Verification items for this drawing (mm, ordinates from the low corner). Give positions to 0.01 mm unless a question says otherwise; leave off trailing zeros. Order: outer loops, then holes, each group sorted by start corner. A loop starts at its lowest first (then second) coordinate and runs counter-clockwise, first axis right, second up.
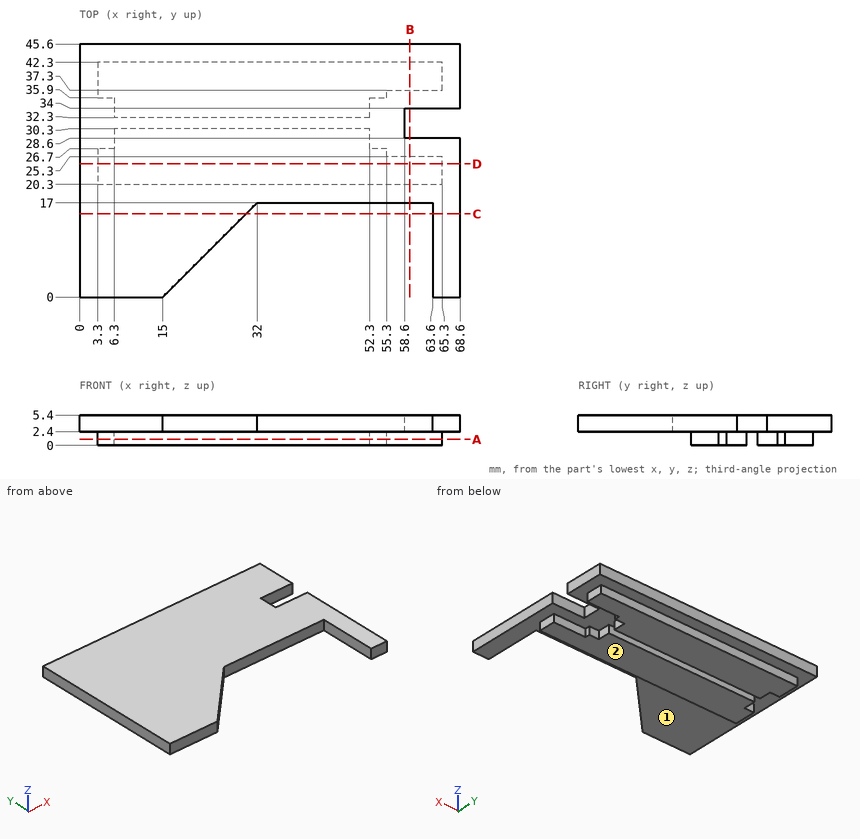
Q1. Release check for a two-part mould opening along Y. For the marked faces 1 and 2 record: pulls with the +Y half, pulls with the -Y half, needs draft (parallel to the pull), parting line crosses it, or undercut.
Q2. Cross-section at D-D, the plane y = 24. Record the boundary of the cut face in (x, z), and give its area (3 significant figures).
Q3. Cross-section at B-B, the plane x = 59.5. Record the boundary of the cut face in (y, z), and give its area (3 significant figures).
Q4. Cross-section at A-A, the plane z = 1.05. Record the boundary of the cut face in (x, y), and give its area (3 significant figures).
Q5. Thickness scan on L1, parallel to Y at x = 44, z = 2.1; L2, parallel to Y at x = 59.5, z = 1.55; L3, parallel to Z at x = 14.5, y = 10.5. Record the ranges inside material, lowest first.
Q6. Cross-section at C-C, the plane y = 15. Record the boundary of the cut face in (x, z), and give its area (3 significant figures).
Q7. Gauge pin test, flat ends, axial feed: P1, Ø8, axis at x = 38.5, y = 15.5, coming from the +Z side; P2, Ø1.2, axis at y = 22.5, z = 1.5, coming from the +X side; P3, Ø1, axis at x = 56, z = 3, coming from the -Y side; P4, Ø0.7, axis at x = 5.5, z = 1, coming from the +Y side. Record the tip position at first contact, or that the pin passes through.
Answers follow:
1. face 1: undercut
1. face 2: needs draft
2. outline: (0, 2.4) - (3.3, 2.4) - (3.3, 0) - (65.3, 0) - (65.3, 2.4) - (68.6, 2.4) - (68.6, 5.4) - (0, 5.4) - close
2. area: 355 mm2
3. outline: (17, 2.4) - (20.3, 2.4) - (20.3, 0) - (25.3, 0) - (25.3, 2.4) - (28.6, 2.4) - (28.6, 5.4) - (17, 5.4) - close; (34, 2.4) - (37.3, 2.4) - (37.3, 0) - (42.3, 0) - (42.3, 2.4) - (45.6, 2.4) - (45.6, 5.4) - (34, 5.4) - close
3. area: 93.6 mm2
4. outline: (3.3, 20.3) - (65.3, 20.3) - (65.3, 25.3) - (55.3, 25.3) - (55.3, 26.7) - (52.3, 26.7) - (52.3, 30.3) - (6.3, 30.3) - (6.3, 26.7) - (3.3, 26.7) - close; (3.3, 35.9) - (6.3, 35.9) - (6.3, 32.3) - (52.3, 32.3) - (52.3, 35.9) - (55.3, 35.9) - (55.3, 37.3) - (65.3, 37.3) - (65.3, 42.3) - (3.3, 42.3) - close
4. area: 1,100 mm2
5. L1: y = 20.3 to 30.3, 32.3 to 42.3
5. L2: y = 20.3 to 25.3, 37.3 to 42.3
5. L3: z = 2.4 to 5.4
6. outline: (0, 2.4) - (30, 2.4) - (30, 5.4) - (0, 5.4) - close; (63.6, 2.4) - (68.6, 2.4) - (68.6, 5.4) - (63.6, 5.4) - close
6. area: 105 mm2
7. P1: stops at z = 5.4
7. P2: stops at x = 65.3
7. P3: stops at y = 17
7. P4: stops at y = 42.3
